Design review of the part built by this model. Coordinates are the model's own, in mm. A direction names the side the tool comes from. Coordinates: 2 decimals unless noted, no trailing zeros.
from build123d import *

# Parameters (mm, degrees)
F2_DEPTH = 12.7
F3_COUNT = 12
F3_ANGLE = 330
F5_D     = 25.4


with BuildPart() as f2:
    # F1 (on Front) → F2 (new body, symmetric)
    with BuildSketch(Plane.XZ):
        with BuildLine():
            Line((0, 27.2142857143), (0, 32.6571428571))
            Line((0, 32.6571428571), (-4.1027982168, 31.163846429))
            Line((-4.1027982168, 31.163846429), (-3.5521770883, 26.9814637274))
            ThreePointArc((-3.5521770883, 26.9814637274), (-1.7798994455, 27.1560178396), (0, 27.2142857143))
        make_face()
        with BuildLine():
            Line((-3.5521770883, 26.9814637274), (-4.1027982168, 31.163846429))
            Line((-4.1027982168, 31.163846429), (-8.4908538679, 29.5667247857))
            ThreePointArc((-8.4908538679, 29.5667247857), (-8.2952422965, 27.7884140488), (-7.8836733992, 26.0473614916))
            ThreePointArc((-7.8836733992, 26.0473614916), (-5.7369683492, 26.6027167992), (-3.5521770883, 26.9814637274))
        make_face()
        with BuildLine():
            Line((-4.1027982168, 31.163846429), (-4.2626125059, 32.3777564729))
            ThreePointArc((-4.2626125059, 32.3777564729), (-6.3710925161, 32.0296450143), (-8.4522905301, 31.5443776985))
            ThreePointArc((-8.4522905301, 31.5443776985), (-8.5050911091, 30.5562048457), (-8.4908538679, 29.5667247857))
            Line((-8.4908538679, 29.5667247857), (-4.1027982168, 31.163846429))
        make_face()
        with BuildLine():
            ThreePointArc((-8.4522905301, 31.5443776985), (-6.3710925161, 32.0296450143), (-4.2626125059, 32.3777564729))
            Line((-4.2626125059, 32.3777564729), (-4.2993944212, 32.6571428571))
            Line((-4.2993944212, 32.6571428571), (-8.3117038653, 32.6571428571))
            ThreePointArc((-8.3117038653, 32.6571428571), (-8.3926831774, 32.1021103437), (-8.4522905301, 31.5443776985))
        make_face()
        with BuildLine():
            Line((-4.1027982168, 31.163846429), (0, 32.6571428571))
            ThreePointArc((0, 32.6571428571), (-2.1358793346, 32.5872214075), (-4.2626125059, 32.3777564729))
            Line((-4.2626125059, 32.3777564729), (-4.1027982168, 31.163846429))
        make_face()
        with BuildLine():
            ThreePointArc((-4.2626125059, 32.3777564729), (-2.1358793346, 32.5872214075), (0, 32.6571428571))
            Line((0, 32.6571428571), (-4.2993944212, 32.6571428571))
            Line((-4.2993944212, 32.6571428571), (-4.2626125059, 32.3777564729))
        make_face()
        with BuildLine():
            ThreePointArc((0, 32.6571428571), (-1.3922286837, 35.486786515), (-3.3594239194, 37.9516043262))
            ThreePointArc((-3.3594239194, 37.9516043262), (-4.1671816864, 37.8714219009), (-4.9730479236, 37.7740492183))
            Line((-4.9730479236, 37.7740492183), (-4.2993944212, 32.6571428571))
            Line((-4.2993944212, 32.6571428571), (0, 32.6571428571))
        make_face()
        with BuildLine():
            Line((-4.2993944212, 32.6571428571), (-4.9730479236, 37.7740492183))
            ThreePointArc((-4.9730479236, 37.7740492183), (-5.7766568393, 37.6595304772), (-6.5776436666, 37.5279176587))
            ThreePointArc((-6.5776436666, 37.5279176587), (-7.661923736, 35.1698741183), (-8.3117038653, 32.6571428571))
            Line((-8.3117038653, 32.6571428571), (-4.2993944212, 32.6571428571))
        make_face()
        with BuildLine():
            ThreePointArc((0.8734905136, 27.2002639925), (0.6971989167, 29.9703946199), (0, 32.6571428571))
            Line((0, 32.6571428571), (0, 27.2142857143))
            ThreePointArc((0, 27.2142857143), (0.4368015242, 27.210780058), (0.8734905136, 27.2002639925))
        make_face()
        with BuildLine():
            ThreePointArc((27.2142857143, 0), (23.1138516304, 14.3654867564), (12.0481915595, 24.4020168651))
            ThreePointArc((12.0481915595, 24.4020168651), (6.8095488061, 19.7367686343), (0, 18.0521428571))
            Line((0, 18.0521428571), (0, 0))
            Line((0, 0), (-2.402809942, 18.2511534992))
            ThreePointArc((-2.402809942, 18.2511534992), (-7.8527791982, 20.3429281496), (-12.0481915595, 24.4020168651))
            ThreePointArc((-12.0481915595, 24.4020168651), (-14.3654867564, -23.1138516304), (27.2142857143, 0))
        make_face()
        with BuildLine():
            ThreePointArc((-7.8836733992, 26.0473614916), (-9.9998299945, 25.3104868981), (-12.0481915595, 24.4020168651))
            ThreePointArc((-12.0481915595, 24.4020168651), (-7.8527791982, 20.3429281496), (-2.402809942, 18.2511534992))
            Line((-2.402809942, 18.2511534992), (-3.5521770883, 26.9814637274))
            ThreePointArc((-3.5521770883, 26.9814637274), (-5.7369683492, 26.6027167992), (-7.8836733992, 26.0473614916))
        make_face()
        with BuildLine():
            Line((0, 18.0521428571), (0, 27.2142857143))
            ThreePointArc((0, 27.2142857143), (-1.7798994455, 27.1560178396), (-3.5521770883, 26.9814637274))
            Line((-3.5521770883, 26.9814637274), (-2.402809942, 18.2511534992))
            ThreePointArc((-2.402809942, 18.2511534992), (-1.2055186491, 18.10198055), (0, 18.0521428571))
        make_face()
        with BuildLine():
            Line((0, 0), (0, 18.0521428571))
            ThreePointArc((0, 18.0521428571), (-1.2055186491, 18.10198055), (-2.402809942, 18.2511534992))
            Line((-2.402809942, 18.2511534992), (0, 0))
        make_face()
        with BuildLine():
            ThreePointArc((0.8734905136, 27.2002639925), (0.4368015242, 27.210780058), (0, 27.2142857143))
            Line((0, 27.2142857143), (0, 18.0521428571))
            ThreePointArc((0, 18.0521428571), (6.8095488061, 19.7367686343), (12.0481915595, 24.4020168651))
            ThreePointArc((12.0481915595, 24.4020168651), (6.6105985846, 26.399191906), (0.8734905136, 27.2002639925))
        make_face()
    extrude(amount=F2_DEPTH, both=True)

    # F3: F2 ×12 about axis
    f3_axis = Axis((0, 0, 0), (0, -1, 0))


with BuildPart() as f2_1:
    add(f2.part)
    for i in range(1, F3_COUNT):
        add(f2.part.rotate(f3_axis, i * F3_ANGLE / (F3_COUNT - 1)))

    # F5 (through all)
    with Locations(Plane.XZ.offset(12.7)):
        with Locations((0, 0)):
            Hole(F5_D / 2)


solid = f2_1.part
Q1. Machinability: for faces 5 (the cylindrical face through (-8.405, -0.178, 32.005)), 6 (the cylindrical face through (28.47, -0.18, 16.56)), 7 (the cylindrical face through (-28.47, -0.18, -16.56)), which of the approach directions +Z, -Z, +X, -X, +Y, -Y give a long, thin tool a straight path to every point of the face, cutting with its end or side? Answer none if there is none.
Q2. The part is to be moulded in two halves that separate along X. For faces 1 (the cylindrical face through (-37.777, -0.178, -4.951)), 2 (the cylindrical face through (-21.568, -0.178, 16.597)), 3 (the cylindrical face through (-0.104, -0.178, 32.935)), 4 (the flat face through (-9, -12.7, -14)), say which applies: pulls with the +X half, pulls with the -X half, needs draft (parallel to the pull), parting line crosses it, or undercut.
Q3. Clearance check with flat-ended pins moving along their axes: pin 1 Ø1 at (x, y) = (9.5, 6) entering from +Z; pin 2 Ø12 at (y, z) = (-2.5, 2.5) entering from -X; pin 3 Ø12 at (y, z) = (9.5, -10.5) entering from -X; pin 4 Ø6 at (x, z) = (-29.5, 26.5) entering from +Y. State where each tip first meets the part, or that it passes through.
Q4. For line 1 (Z direction, x = 29.5, y = 9); line 2 (X direction, y = -7, z = 27.5); line 3 (Z direction, x = 25, y = -4.5), list the stretches that pass through material, from the lowest coordinate up.
Entries:
1. face 5: +Y, -Y
1. face 6: +X, +Y, -Y
1. face 7: -X, +Y, -Y
2. face 1: pulls with the -X half
2. face 2: undercut
2. face 3: undercut
2. face 4: needs draft
3. pin 1: stops at z = 33.41
3. pin 2: stops at x = -37.95
3. pin 3: stops at x = -37.83
3. pin 4: passes through
4. line 1: z = -16.49 to -7.26, -0.76 to 8.49, 18.01 to 24.11
4. line 2: x = -24.35 to -15.47, -8.24 to 0.88, 6.47 to 16.17
4. line 3: z = -15.34 to 10.75, 13.44 to 23.82
